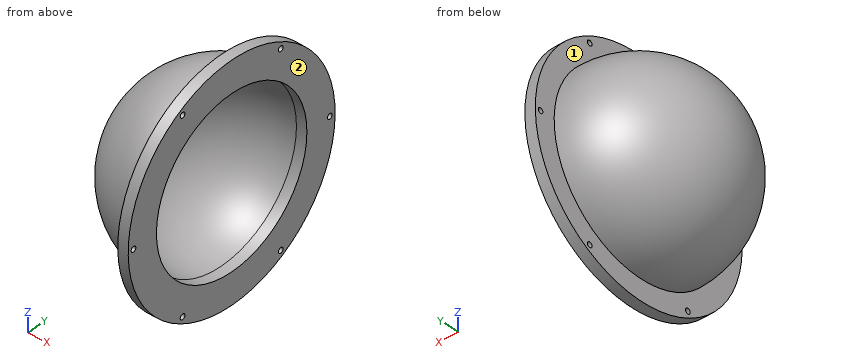
```python
from build123d import *

# Parameters (mm, degrees)
SKETCH_4_R               = 1.25
CUT_EXTRUDE_1_DEPTH      = 6
PATTERN_CIRCULAR_1_COUNT = 6


with BuildPart() as part:
    # 草图2 → 旋转1 (revolve)
    with BuildSketch(Plane(origin=(0, 0, 0), x_dir=(1, 0, 0), z_dir=(0, 1, 0))):
        with BuildLine():
            Line((-45, 0), (-50, 0))
            ThreePointArc((-50, 0), (-36.819805153, 31.819805153), (-5, 45))
            Line((-5, 45), (-5, 55))
            Line((-5, 55), (0, 55))
            Line((0, 55), (0, 40))
            Line((0, 40), (-5, 40))
            ThreePointArc((-5, 40), (-33.284271247, 28.284271247), (-45, 0))
        make_face()
    revolve(axis=Axis((95.822015525, 0, 0), (-1, 0, 0)))

    # 草图4 → 切除-拉伸1 (cut, through all)
    with BuildSketch(Plane.ZY.offset(5)):
        with Locations((0, 52.2)):
            Circle(SKETCH_4_R)
    cut_extrude_1 = extrude(amount=-CUT_EXTRUDE_1_DEPTH, mode=Mode.SUBTRACT)

    # 阵列(圆周)1: 切除-拉伸1 ×6 about axis
    pattern_circular_1_axis = Axis((0, 0, 0), (1, 0, 0))
    for i in range(1, PATTERN_CIRCULAR_1_COUNT):
        add(cut_extrude_1.rotate(pattern_circular_1_axis, i * 360 / PATTERN_CIRCULAR_1_COUNT), mode=Mode.SUBTRACT)


solid = part.part
```
Can you work these out from the model? Positions are in its coordinate system, mm. Face numbers are marked on the shaded views. A direction names the side the tool comes from. Coordinates: 2 decimals unless noted, no trailing zeros. Loops run counter-clockwise (first coordinate to the right, second up) from the corner with the lowest first, then second, coordinate; pieces in that order, holes last.
1) Imagine slicing it at C-C on x = -28. List the corners of the cut face in (y, z) for me, plus the area to 3 significant figures.
2) Imagine slicing it at A-A on y = 0. List the corners of the cut face in (x, z) for me.
3) Which directions (+Z, -Z, +X, -X, +Y, -Y) give clear straight access to the entire face, cutting with the end or side of a thin tool? Please do the marked faces 1 and 2.
4) I need wall thicknesses on probe 1 along Y at (x, z) = (-3, 0); probe 2 along Z at (x, y) = (-3.45, 0); probe 3 along X at (y, z) = (-24.5, -39.5). Which ranges of each line are inside material? Lowest first, please.
5) For pin 1 (10 mm diameter, centred on y = 40, z = -33, fed in from -X); pin 2 (2 mm diameter, centred on y = 39, z = -3.5, fed in from -X); pin 3 (1.5 mm diameter, centred on x = -6, z = -37, fed in from -Y), each with a flat end and sliding along its axis, tell me the tip position at first contact or that it passes through.
6) Imagine slicing it at B-B on z = -23. List the corners of the cut face in (x, y) for me.
Completed:
1. outline: circle Ø77.36 at (0, 0); hole circle Ø65.45 at (0, 0)
1. area: 1,340 mm2
2. outline: (-5, -55) - (0, -55) - (0, -40) - (-5, -40) arc R40 cw to (-5, 40) - (0, 40) - (0, 55) - (-5, 55) - (-5, 45) arc R45 ccw to (-5, -45) - close
3. face 1: -X
3. face 2: +Z, -Z, +X, +Y, -Y
4. probe 1: y = -55 to -53.45, -50.95 to -40, 40 to 50.95, 53.45 to 55
4. probe 2: z = -55 to -40, 40 to 55
4. probe 3: x = -5 to 0
5. pin 1: stops at x = -5
5. pin 2: stops at x = -28.86
5. pin 3: stops at y = -26.65
6. outline: (-5, -49.96) - (0, -49.96) - (0, -32.73) - (-5, -32.73) arc R32.73 cw to (-5, 32.73) - (0, 32.73) - (0, 49.96) - (-5, 49.96) - (-5, 38.68) arc R38.68 ccw to (-5, -38.68) - close
